Part model, mm, in its own coordinate system. A direction names the side the tool comes from. Coordinates: 2 decimals unless noted, no trailing zeros. Order: outer loops, then holes, each group sorted by start corner. A loop starts at its lowest first (then second) coordinate and runs counter-clockwise, first axis right, second up.
from build123d import *

# Parameters (mm, degrees)
SALIENTE_EXTRUIR1_DEPTH = 30
CROQUIS3_R              = 2.475
CORTAR_EXTRUIR1_DEPTH   = 287.780312831
CROQUIS4_R              = 1.5
CORTAR_EXTRUIR2_DEPTH   = 191.467453482
CROQUIS5_W              = 45
CROQUIS5_H              = 30
SALIENTE_EXTRUIR2_DEPTH = 12
CORTAR_EXTRUIR3_DEPTH   = 203.637632672
CROQUIS7_R              = 1.5
CORTAR_EXTRUIR4_DEPTH   = 184.243021226


with BuildPart() as part:
    # Croquis1 → Saliente-Extruir1 (new body)
    with BuildSketch(Plane.XY):
        with BuildLine():
            Line((-22.5, -5), (22.5, -5))
            ThreePointArc((22.5, -5), (34.627023925, -7.412215038), (44.90781839, -14.28162228))
            Line((44.90781839, -14.28162228), (115.618496509, -84.992300399))
            Line((115.618496509, -84.992300399), (115.618496509, -134.992300399))
            Line((115.618496509, -134.992300399), (125.618496509, -134.992300399))
            Line((125.618496509, -134.992300399), (125.618496509, -80.850164775))
            Line((125.618496509, -80.850164775), (122.689564321, -77.921232587))
            Line((122.689564321, -77.921232587), (51.978886202, -7.210554468))
            ThreePointArc((51.978886202, -7.210554468), (38.453858249, 1.826580287), (22.5, 5))
            Line((22.5, 5), (-22.5, 5))
            ThreePointArc((-22.5, 5), (-38.453858249, 1.826580287), (-51.978886202, -7.210554468))
            Line((-51.978886202, -7.210554468), (-122.689564321, -77.921232587))
            Line((-122.689564321, -77.921232587), (-125.618496509, -80.850164775))
            Line((-125.618496509, -80.850164775), (-125.618496509, -134.992300399))
            Line((-125.618496509, -134.992300399), (-115.618496509, -134.992300399))
            Line((-115.618496509, -134.992300399), (-115.618496509, -84.992300399))
            Line((-115.618496509, -84.992300399), (-44.90781839, -14.28162228))
            ThreePointArc((-44.90781839, -14.28162228), (-34.627023925, -7.412215038), (-22.5, -5))
        make_face()
    extrude(amount=SALIENTE_EXTRUIR1_DEPTH)

    # Croquis3 → Cortar-Extruir1 (cut, through all)
    with BuildSketch(Plane.ZY.offset(125.618496509)):
        with Locations((15, -124.992300399)):
            Circle(CROQUIS3_R)
    extrude(amount=-CORTAR_EXTRUIR1_DEPTH, mode=Mode.SUBTRACT)

    # Croquis4 → Cortar-Extruir2 (cut, through all)
    with BuildSketch(Plane(origin=(0, 5, 0), x_dir=(1, 0, 0), z_dir=(0, 1, 0))):
        with Locations(Location((0, -15, 0), (0, 0, 270))):
            Circle(CROQUIS4_R)
        with Locations(Location((18, -15, 0), (0, 0, 270))):
            Circle(CROQUIS4_R)
        with Locations(Location((-18, -15, 0), (0, 0, 270))):
            Circle(CROQUIS4_R)
    extrude(amount=-CORTAR_EXTRUIR2_DEPTH, mode=Mode.SUBTRACT)

    # Croquis5 → Saliente-Extruir2 (add)
    with BuildSketch(Plane(origin=(0, 5, 0), x_dir=(1, 0, 0), z_dir=(0, 1, 0))):
        with Locations((0, -15)):
            Rectangle(CROQUIS5_W, CROQUIS5_H)
    extrude(amount=SALIENTE_EXTRUIR2_DEPTH)

    # Croquis6 → Cortar-Extruir3 (cut, through all)
    with BuildSketch(Plane(origin=(22.5, 0, 0), x_dir=(0, 0, -1), z_dir=(1, 0, 0))):
        Polygon((0, 5), (-30, 8.47111843), (-30, 19.923097654), (0, 19.923097654), align=None)
    extrude(amount=-CORTAR_EXTRUIR3_DEPTH, mode=Mode.SUBTRACT)

    # Croquis7 → Cortar-Extruir4 (cut, through all)
    with BuildSketch(Plane.XZ.offset(5)):
        with Locations(Location((0, 15, 0), (0, 0, 90))):
            Circle(CROQUIS7_R)
        with Locations(Location((-18, 15, 0), (0, 0, 90))):
            Circle(CROQUIS7_R)
        with Locations(Location((18, 15, 0), (0, 0, 90))):
            Circle(CROQUIS7_R)
    extrude(amount=-CORTAR_EXTRUIR4_DEPTH, mode=Mode.SUBTRACT)


solid = part.part
Q1. Cut at D-D on x = -48. Write the cut outline in (y, z), and give its area (3 significant figures).
Results list:
outline: (-17.37, 0) - (-3.71, 0) - (-3.71, 30) - (-17.37, 30) - close
area: 410 mm2
Q2. Which spindle directions (+Z, -Z, +X, -X, +Y, -Y) get a long thin tool onto all of the face, cutting with end or side? Do faces 1 (the face through (-120.688, -127.408, 14.463)), 2 (the face through (-34.79, -7.48, 14.79)). Say none if no direction does.
Results list:
face 1: +X, -X
face 2: +Z, -Z, -Y
Q3. Pin check, flat tips, straight feed: pin 1 Ø3 at (y, z) = (7.5, 11) entering from +X; pin 2 Ø1.5 at (y, z) = (-30.5, 14) entering from -X; pin 3 Ø4 at (x, y) = (-72, -42.5) entering from +Z; pin 4 Ø4 at (y, z) = (-55, 12.5) entering from +X. Stop position of each tip, or through.
Results list:
pin 1: stops at x = 22.5
pin 2: stops at x = -76.02
pin 3: stops at z = 30
pin 4: stops at x = 101.77
Q4. Mould opens along X. For faces 3 (the face through (34.466, -7.346, 14.79)), 4 (the face through (-1, -3, 0)), 5 (the face through (-38.242, 1.914, 14.79)) say: pulls with the +X half, pulls with the -X half, needs draft (parallel to the pull), parting line crosses it, or undercut.
Results list:
face 3: undercut
face 4: needs draft
face 5: pulls with the -X half
Q5. Cut at A-A on y = -105. Write the cut outline in (x, z), and give its area (3 significant figures).
Results list:
outline: (-125.62, 0) - (-115.62, 0) - (-115.62, 30) - (-125.62, 30) - close; (115.62, 0) - (125.62, 0) - (125.62, 30) - (115.62, 30) - close
area: 600 mm2
Q6. Wall check: line 1 along X through (y, z) = (-97, 10); line 2 along Z through (x, y) = (-18, 0); line 3 along X through (y, z) = (0.5, 15). Give the ranges that are in metal, low to high.
Results list:
line 1: x = -125.62 to -115.62, 115.62 to 125.62
line 2: z = 0 to 13.5, 16.5 to 30
line 3: x = -41.34 to -19.5, -16.5 to -1.5, 1.5 to 16.5, 19.5 to 41.34
Q7. Cut at C-C on z = 6.25. Write the cut outline in (x, y), and give its area (3 significant figures).
Results list:
outline: (-125.62, -134.99) - (-115.62, -134.99) - (-115.62, -84.99) - (-44.91, -14.28) arc R31.69 cw to (-22.5, -5) - (22.5, -5) arc R31.69 cw to (44.91, -14.28) - (115.62, -84.99) - (115.62, -134.99) - (125.62, -134.99) - (125.62, -80.85) - (51.98, -7.21) arc R41.69 ccw to (22.5, 5) - (22.5, 5.72) - (-22.5, 5.72) - (-22.5, 5) arc R41.69 ccw to (-51.98, -7.21) - (-125.62, -80.85) - close
area: 4,140 mm2
Q8. Cut at B-B on z = 20.5. Write the cut outline in (x, y), and give its area (3 significant figures).
Results list:
outline: (-125.62, -134.99) - (-115.62, -134.99) - (-115.62, -84.99) - (-44.91, -14.28) arc R31.69 cw to (-22.5, -5) - (22.5, -5) arc R31.69 cw to (44.91, -14.28) - (115.62, -84.99) - (115.62, -134.99) - (125.62, -134.99) - (125.62, -80.85) - (51.98, -7.21) arc R41.69 ccw to (22.5, 5) - (22.5, 7.37) - (-22.5, 7.37) - (-22.5, 5) arc R41.69 ccw to (-51.98, -7.21) - (-125.62, -80.85) - close
area: 4,220 mm2
